Verification items for this drawing (mm, ordinates from the low corner). A direction names the side the tool comes from. Coordinates: 2 decimals unless noted, no trailing zeros. Write each loop counter-clockwise with the first axis right and the second up, starting at its lowest first coordinate (ties: lowest second). Pieces come first, ordered by that corner, then holes. Notation, with made-up numbers: M -16,39.25 L 23,39.25 A20 ccw 23,66.25 Z; hole C 86,9.25 d8. An arc over 180 degrees is marked long. Put each result on its own line as item: value. Start each with the question number.
1) Cross-section at C-C on z = 6.75. Record the cut outline in (x, y).
2) Cross-section at A-A on y = 7. Record the cut outline in (x, z) (1 decimal).
3) Scan lines: line 1 along Y through (x, z) = (0.75, 3.5) (1 decimal); line 2 along Z through (x, y) = (3, 10) (1 decimal); line 3 along X through (y, z) = (3.5, 3) (1 decimal). Record each from-to range of solid material in increasing order.
4) Gauge pin test, flat ends, axial feed: pin 1 (1.7 mm diameter, centred on x = 4, z = 5, fed in from -Y) (1 decimal); pin 2 (1 mm diameter, centred on x = 5.5, y = 11, fed in from -Z) (1 decimal); pin 3 (3.5 mm diameter, centred on x = 5, z = 5, fed in from -Y). Record the tip position at first contact, or that the pin passes through.
5) Cross-section at B-B on x = 1. Count the separate pieces of the cut face and the enclosed holes in it, plus the area to 3 significant figures.
6) Cross-section at D-D on y = 1.75. Record the cut outline in (x, z).
7) Set-up check for the marked faces 4, 5, 6 and 7: record each of +Z, -Z, +X, -X, +Y, -Y from which the full face is reachable in a straight line by a thin tool's end or side.
8) Mould release check, pull along Y, two halves, no side actions. Record for the marked faces 1, 2 and 3: released by +Y, released by -Y, zero draft, split by the parting line, or undercut.
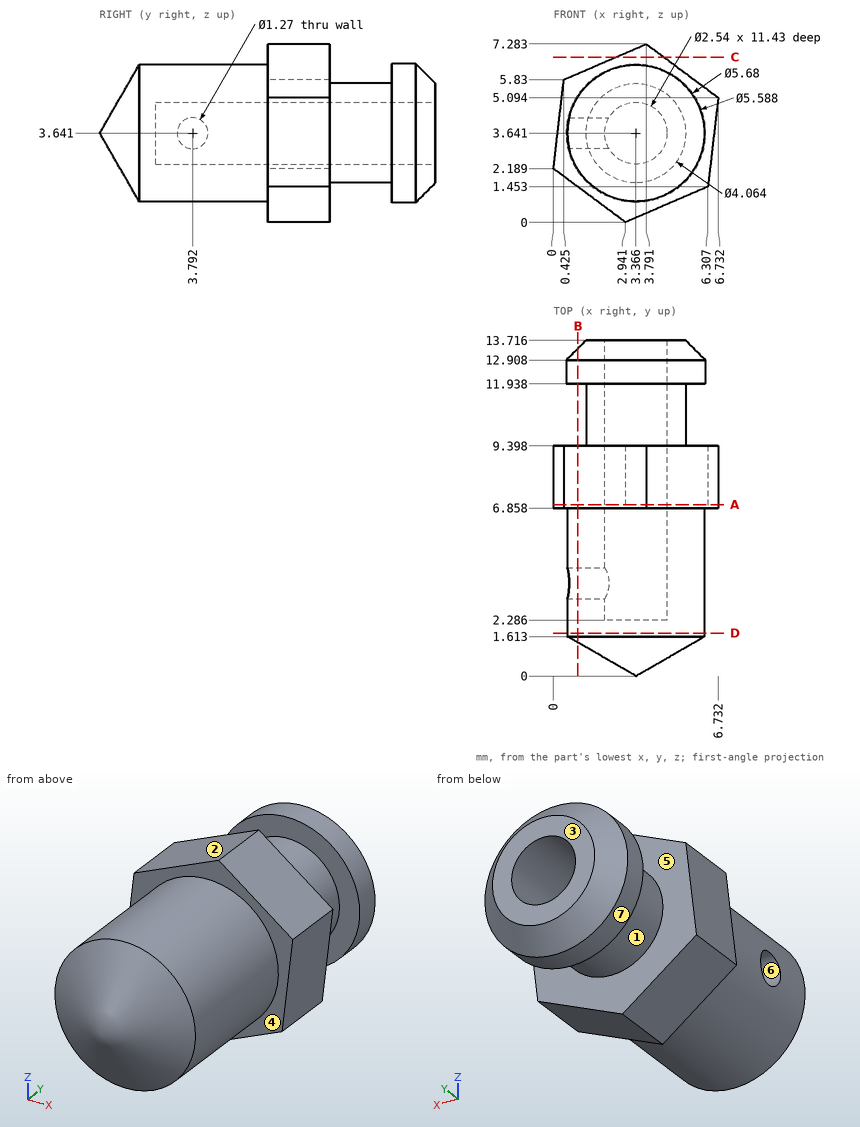
Answer key:
1. outline: M 2.56,6.86 L 4.51,6.86 L 4.51,9.4 L 2.56,9.4 Z
2. outline: M 0,2.2 L 2.9,0 L 6.3,1.5 L 6.7,5.1 L 3.8,7.3 L 0.4,5.8 Z; hole C 3.4,3.6 d2.5
3. line 1: y = 1.5 to 3.2, 4.4 to 9.4, 11.9 to 13.1
3. line 2: z = 1.6 to 2.4, 4.9 to 5.6
3. line 3: x = 0.6 to 2.3, 4.5 to 6.1
4. pin 1: stops at y = 0.4
4. pin 2: stops at z = 2.4
4. pin 3: stops at y = 0.22
5. separate pieces: 2
5. enclosed holes: 1
5. area: 30.6 mm²
6. outline: C 3.37,3.64 d5.59
7. face 4: -Y
7. face 5: none
7. face 6: -X
7. face 7: +Y
8. face 1: undercut
8. face 2: zero draft
8. face 3: released by +Y
